Design review of the part built by this model. Coordinates are the model's own, in mm. Face numbers are marked on the shaded views. A direction names the side the tool comes from. Give positions to 0.01 mm unless a question says otherwise; leave off trailing zeros. Loops run counter-clockwise (first coordinate to the right, second up) from the corner with the lowest first, then second, coordinate; pieces in that order, holes last. Notation, with made-up numbers: (56, 81.25) -> (114, 81.25) arc R9 cw to (114, 98.25) -> close; hole circle Ø10 at (67, -7). An arc over 180 degrees is marked (long way). Answer in a Markdown table with one row per item. Add a question column.
(1) Consider section D-D on y = 23.5. Write out the cut boundary in (x, z), then the cut area to 3 significant figures.
(2) For the marked faces 4 and 5, list the 3-axis set-ups (+Z, -Z, +X, -X, +Y, -Y) from which the entire face can be reached by the end or side of a thin tool; tool diameter is ignored.
(3) Consider section A-A on x = 0. Write out the cut boundary in (y, z).
(4) For line 1 (X direction, y = 20.5, z = 1); line 2 (Z direction, x = 20, y = 12.5); line 3 (Y direction, x = 0, z = 2.95), list the stretches that pass through material, from the lowest coordinate up.
(5) Consider section B-B on y = 0. Write out the cut boundary in (x, z).
(6) Draft analysis for pull direction Y (two halves, no side actions). For the marked faces 1, 2 and 3, state which applies: +Y half, -Y half, draft (parallel to the pull), parting line (faces both ways), or undercut.
(7) Consider section C-C on z = 2.25. Write out the cut boundary in (x, y), then the cut area to 3 significant figures.
(8) For pin 1 (1 mm diameter, centred on y = 8.5, z = 7, fed in from -X); pin 2 (5 mm diameter, centred on y = -4.5, z = 9.5, fed in from -X); pin 3 (5 mm diameter, centred on y = 1, z = 11, fed in from +X), all flat-tipped, find the tip position at first contact; note any pin that passes through.
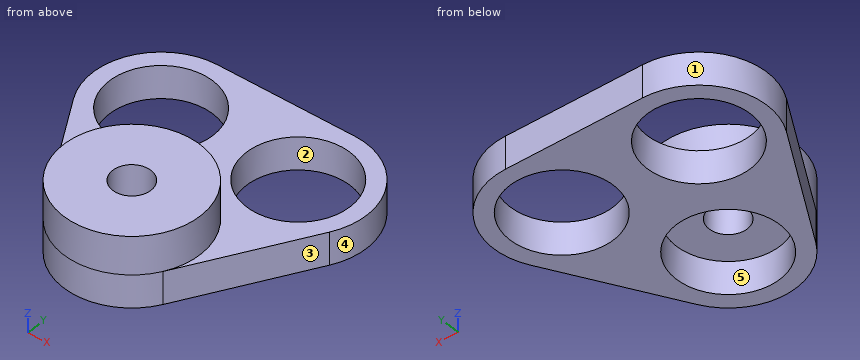
from build123d import *

# Parameters (mm, degrees)
CROQUIS1_R              = 9.5
SALIENTE_EXTRUIR1_DEPTH = 6
CROQUIS2_R              = 12.5
CROQUIS2_R_2            = 3.5
SALIENTE_EXTRUIR3_DEPTH = 7


with BuildPart() as part:
    # Croquis1 → Saliente-Extruir1 (new body)
    with BuildSketch(Plane.XY):
        with BuildLine():
            Line((-23.325317547, 15.400635095), (-10.825317547, -6.25))
            ThreePointArc((-10.825317547, -6.25), (0, -12.5), (10.825317547, -6.25))
            Line((10.825317547, -6.25), (23.325317547, 15.400635095))
            ThreePointArc((23.325317547, 15.400635095), (23.325317547, 27.900635095), (12.5, 34.150635095))
            Line((12.5, 34.150635095), (-12.5, 34.150635095))
            ThreePointArc((-12.5, 34.150635095), (-23.325317547, 27.900635095), (-23.325317547, 15.400635095))
        make_face()
        Circle(CROQUIS1_R, mode=Mode.SUBTRACT)
        with Locations((12.5, 21.650635095)):
            Circle(CROQUIS1_R, mode=Mode.SUBTRACT)
        with Locations((-12.5, 21.650635095)):
            Circle(CROQUIS1_R, mode=Mode.SUBTRACT)
    extrude(amount=SALIENTE_EXTRUIR1_DEPTH)

    # Croquis2 → Saliente-Extruir3 (add)
    with BuildSketch(Plane.XY.offset(6)):
        with Locations(Location((0, 0, 0), (0, 0, 210))):
            Circle(CROQUIS2_R)
        Circle(CROQUIS2_R_2, mode=Mode.SUBTRACT)
    extrude(amount=SALIENTE_EXTRUIR3_DEPTH)


solid = part.part
Values follow:
| question | item | result |
|---|---|---|
| 1 | outline | (-24.86, 0) -> (-21.82, 0) -> (-21.82, 6) -> (-24.86, 6) -> close; (-3.18, 0) -> (3.18, 0) -> (3.18, 6) -> (-3.18, 6) -> close; (21.82, 0) -> (24.86, 0) -> (24.86, 6) -> (21.82, 6) -> close |
| 1 | area | 74.7 mm2 |
| 2 | face 4 | +Z, -Z, +X |
| 2 | face 5 | -Z |
| 3 | outline | (-12.5, 0) -> (-9.5, 0) -> (-9.5, 6) -> (-3.5, 6) -> (-3.5, 13) -> (-12.5, 13) -> close; (3.5, 6) -> (9.5, 6) -> (9.5, 0) -> (34.15, 0) -> (34.15, 6) -> (12.5, 6) -> (12.5, 13) -> (3.5, 13) -> close |
| 4 | line 1 | -24.95 to -21.93, -3.07 to 3.07, 21.93 to 24.95 |
| 4 | line 2 | 0 to 6 |
| 4 | line 3 | -12.5 to -9.5, 9.5 to 34.15 |
| 5 | outline | (-14.43, 0) -> (-9.5, 0) -> (-9.5, 6) -> (-3.5, 6) -> (-3.5, 13) -> (-12.5, 13) -> (-12.5, 6) -> (-14.43, 6) -> close; (3.5, 6) -> (9.5, 6) -> (9.5, 0) -> (14.43, 0) -> (14.43, 6) -> (12.5, 6) -> (12.5, 13) -> (3.5, 13) -> close |
| 6 | face 1 | parting line |
| 6 | face 2 | undercut |
| 6 | face 3 | -Y half |
| 7 | outline | (-23.33, 15.4) -> (-10.83, -6.25) arc R12.5 ccw to (10.83, -6.25) -> (23.33, 15.4) arc R12.5 ccw to (12.5, 34.15) -> (-12.5, 34.15) arc R12.5 ccw to start; hole circle Ø19 at (-12.5, 21.65); hole circle Ø19 at (0, 0); hole circle Ø19 at (12.5, 21.65) |
| 7 | area | 848 mm2 |
| 8 | pin 1 | x = -9.6 |
| 8 | pin 2 | x = -12.34 |
| 8 | pin 3 | x = 12.5 |
